Print and shaded views of the part. All mm, measured from the part's lowest x, y and z. A direction names the side the tool comes from. Round coordinates to 2 decimals unless told otherwise and drop trailing zeros. Write each loop counter-clockwise with the first axis right and the second up, starting at its lowest first coordinate (ties: lowest second). Pieces come first, ordered by that corner, then holes. Notation, with made-up numbers: (-5.5, 21) - (37.5, 21) arc R9 cw to (37.5, 38) - close; hole circle Ø5 at (-10, 64.5). An arc over 180 degrees is marked (long way). Answer as a JSON object with one key per item and string values. Group by question number.
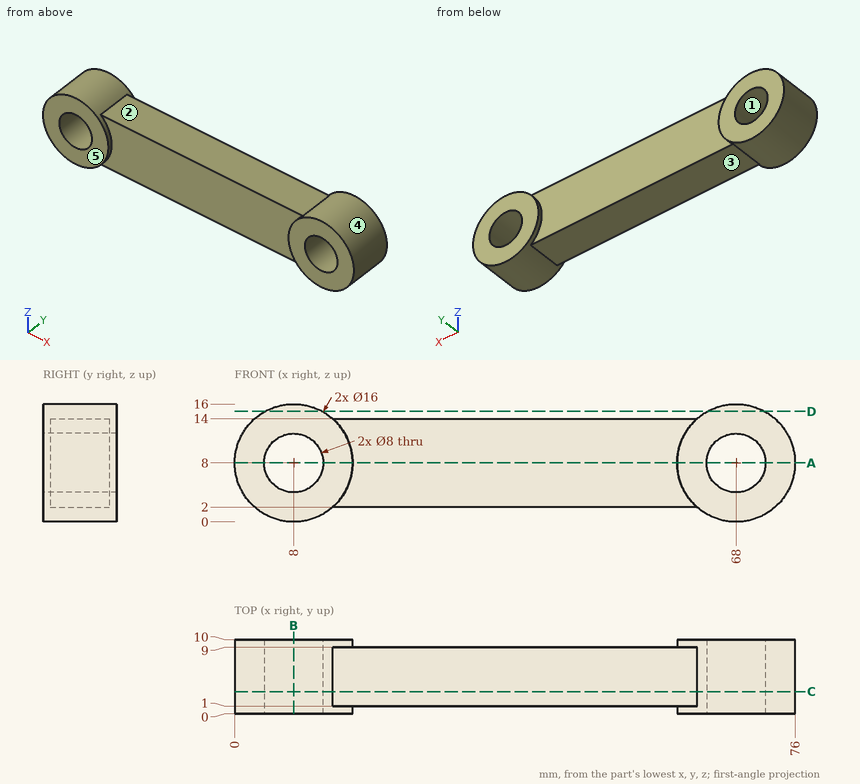
(1) Slice it at D-D (z = 15). Write the cut outline in (x, y), then the cut area to 3 significant figures.
(2) 3-axis set-ups, long thin cutter, end or side, ignore diameter. For the marked faces 1, 2 and 3: which of +Z, -Z, +X, -X, +Y, -Y reach the whole face in a straight line?
(3) Slice it at A-A (z = 8). Write the cut outline in (x, y).
(4) Slice it at C-C (y = 3). Write the cut outline in (x, z), then the cut area to 3 significant figures.
(5) Pull direction X, two halves, no side cores. Call the marked faces 4 and 5: pulls with the +X half, pulls with the -X half, needs draft (parallel to the pull), parting line crosses it, or undercut.
(6) Slice it at B-B (x = 8). Write the cut outline in (y, z), then the cut area to 3 significant figures.
(7) Flat gauge pins, fed straight in: pin 1 (1 mm diameter, centred on x = 19.5, z = 6.5, fed in from +Y); pin 2 (5 mm diameter, centred on x = 54, y = 1.5, fed in from +Z); pin 3 (3 mm diameter, centred on y = 1.5, z = 13.5, fed in from +X). Where does each tip first touch, or does it go through?
(8) Drill centre lines: line 1 (X direction, y = 3.5, z = 8); line 2 (Z direction, x = 8, y = 7.75); line 3 (X direction, y = 3.5, z = 9.75). Where is each one in solid material? Low to high. Write a range as from..to.
Answer:
{
 "1": {"outline": "(4.13, 0) - (11.87, 0) - (11.87, 10) - (4.13, 10) - close; (64.13, 0) - (71.87, 0) - (71.87, 10) - (64.13, 10) - close", "area": "155 mm²"},
 "2": {"face 1": "+Y, -Y", "face 2": "+Z, +Y, -Y", "face 3": "-Z, +Y, -Y"},
 "3": {"outline": "(0, 0) - (4, 0) - (4, 10) - (0, 10) - close; (12, 0) - (16, 0) - (16, 1) - (60, 1) - (60, 0) - (64, 0) - (64, 10) - (60, 10) - (60, 9) - (16, 9) - (16, 10) - (12, 10) - close; (72, 0) - (76, 0) - (76, 10) - (72, 10) - close"},
 "4": {"outline": "(13.29, 2) - (62.71, 2) arc R8 ccw (long way) to (62.71, 14) - (13.29, 14) arc R8 ccw (long way) to start; hole circle Ø8 at (8, 8); hole circle Ø8 at (68, 8)", "area": "850 mm²"},
 "5": {"face 4": "undercut", "face 5": "needs draft"},
 "6": {"outline": "(0, 0) - (10, 0) - (10, 4) - (0, 4) - close; (0, 12) - (10, 12) - (10, 16) - (0, 16) - close", "area": "80.0 mm²"},
 "7": {"pin 1": "y = 9", "pin 2": "z = 14", "pin 3": "x = 74.93"},
 "8": {"line 1": "0..4, 12..64, 72..76", "line 2": "0..4, 12..16", "line 3": "0.19..4.4, 11.6..64.4, 71.6..75.81"}
}
